from build123d import *

# Parameters (mm, degrees)
CYLINDER_R           = 2.15
CYLINDER_DEPTH       = 50
CYLINDER_PITCH_ANGLE = 90
BOX002_W             = 14
BOX002_H             = 11
BOX002_DEPTH         = 20.5
CHAMFER_SIZE         = 4
FILLET001_R          = 5
BOX003_W             = 14
BOX003_H             = 25
BOX003_DEPTH         = 4
BOX003_ROLL_ANGLE    = -15
BOX004_W             = 14
BOX004_H             = 2.5
BOX004_DEPTH         = 5
POCKET006_DEPTH      = 15


with BuildPart() as cylinder:
    # Cylinder → Cylinder (new body)
    with BuildSketch(Plane.XY):
        Circle(CYLINDER_R)
    extrude(amount=CYLINDER_DEPTH)


with BuildPart() as cylinder_1:
    # Cylinder pitch: moved
    add(cylinder.part.rotate(Axis((0, 0, 0), (0, 1, 0)), CYLINDER_PITCH_ANGLE))


with BuildPart() as cylinder_2:
    # Cylinder placement: moved
    add(cylinder_1.part.moved(Location((31, -6, 12.9))))


with BuildPart() as fillet001:
    # Box002 → Box002 (new body)
    with BuildSketch(Plane(origin=(52, -12, -3), x_dir=(1, 0, 0), z_dir=(0, 0, 1))):
        with Locations((7, 5.5)):
            Rectangle(BOX002_W, BOX002_H)
    extrude(amount=BOX002_DEPTH)

    # Chamfer
    chamfer_edges = [fillet001.edges().sort_by_distance(p)[0] for p in [
        (59, -1, -3),
    ]]
    chamfer(chamfer_edges, length=CHAMFER_SIZE)

    # Fillet001
    fillet001_edges = [fillet001.edges().sort_by_distance(p)[0] for p in [
        (59, -1, 17.5),
    ]]
    fillet(fillet001_edges, radius=FILLET001_R)


with BuildPart() as cube002:
    # Box003 → Box003 (new body)
    with BuildSketch(Plane.XY):
        with Locations((7, 12.5)):
            Rectangle(BOX003_W, BOX003_H)
    extrude(amount=BOX003_DEPTH)


with BuildPart() as cube002_1:
    # Box003 roll: moved
    add(cube002.part.rotate(Axis((0, 0, 0), (1, 0, 0)), BOX003_ROLL_ANGLE))


with BuildPart() as cube002_2:
    # Box003 placement: moved
    add(cube002_1.part.moved(Location((52, -12, -3))))


with BuildPart() as obj1:
    # Box004 → Box004 (new body)
    with BuildSketch(Plane(origin=(52, -12, 14), x_dir=(1, 0, 0), z_dir=(0, 0, 1))):
        with Locations((7, 1.25)):
            Rectangle(BOX004_W, BOX004_H)
    extrude(amount=BOX004_DEPTH)

    # Fusion: union Fillet001, Cube002
    add(fillet001.part)
    add(cube002_2.part)

    # Cut001: cut Cylinder
    add(cylinder_2.part, mode=Mode.SUBTRACT)

    # Sketch006 → Pocket006 (cut)
    with BuildSketch(Plane.YZ.offset(66)):
        Polygon((13.183422, -5.606773), (-4.041064, -0.991486), (-0.407217, 12.570217), align=None)
    extrude(amount=-POCKET006_DEPTH, mode=Mode.SUBTRACT)


solid = obj1.part
The listing builds one solid part. Answer for the finished solid, in the listing's coordinates (mm). A direction names the side the tool comes from. Coordinates: 2 decimals unless noted, no trailing zeros. Loops run counter-clockwise (first coordinate to the right, second up) from the corner with the lowest first, then second, coordinate; pieces in that order, holes last.
1) Find section B-B on z = 12.9. Write down the section's boundary in (x, y), then the cut area to 3 significant figures.
2) Flat-ended cylindrical pins translate along their axes: pin 1 Ø5 at (x, y) = (62, -5) entering from -Z; pin 2 Ø3 at (x, z) = (64, 9.5) entering from +Y; pin 3 Ø1.6 at (x, z) = (56, 18.5) entering from +Y. Find the tip coordinate at first contact, or state that the pin passes through.
3) Find section D-D on z = 3.75. Write down the section's boundary in (x, y).
4) Find section A-A on x = 64.25. Write down the section's boundary in (y, z).
5) Find the intervals of material crossed by L1, parallel to Y at x = 53, z = 14; L2, parallel to Z at x = 64, y = -7.5; L3, parallel to Y at x = 60.5, z = 12.9, in increasing order.
6) Find section C-C on y = -2.5. Write down the section's boundary in (x, z).
7) A tool of negligible diameter and unlimited length cuts with its end or side. For faces 1 (the face through (59, -8, 17.5)), 2 (the face through (58.902, -7.308, 14.606)), 3 (the face through (59.098, -2.542, 4.604)), from which of +Z, -Z, +X, -X, +Y, -Y can it reach the whole face along a straight path? Write none if from no direction.
Values:
1. outline: (52, -12) - (66, -12) - (66, -8.15) - (52, -8.15) - close; (52, -3.85) - (66, -3.85) - (66, -1.02) - (52, -1.02) - close
1. area: 93.6 mm2
2. pin 1: stops at z = -5.55
2. pin 2: stops at y = -1
2. pin 3: stops at y = -9.5
3. outline: (52, -12) - (66, -12) - (66, -2.77) - (52, -2.77) - close
4. outline: (-12, -3) - (12.15, -9.47) - (13.18, -5.61) - (-4.04, -0.99) - (-1, 10.36) - (-1, 12.5) arc R5 ccw to (-6, 17.5) - (-9.5, 17.5) - (-9.5, 19) - (-12, 19) - close; hole circle Ø4.3 at (-6, 12.9)
5. L1: y = -12 to -7.85, -4.15 to -1.23
5. L2: z = -4.21 to 11.36, 14.44 to 17.5
5. L3: y = -12 to -8.15, -3.85 to -1.02
6. outline: (52, -5.55) - (66, -5.55) - (66, -1.4) - (52, -1.4) - close; (52, 4.76) - (66, 4.76) - (66, 16.07) - (52, 16.07) - close
7. face 1: +Z, +X, -X, +Y
7. face 2: +X, -X
7. face 3: +X, -X, +Y
